Build history of the part. All positions in model axes, mm. Face numbers are marked on the shaded views. A direction names the side the tool comes from. Round coordinates to 2 decimals unless told otherwise and drop trailing zeros. Write each loop counter-clockwise with the first axis right and the second up, starting at its lowest first coordinate (ties: lowest second). Pieces come first, ordered by that corner, then holes. Notation, with made-up numbers: (45, 38) -> (73, 38) arc R21 ccw to (73, 69) -> close; hole circle Ø11 at (-13.5, -8.75). An arc over 180 degrees is marked (long way). Answer in a Markdown table with one row per item.
```python
from build123d import *

# Parameters (mm, degrees)
SKETCH2_W           = 130
SKETCH2_H           = 130
BOSS_EXTRUDE1_DEPTH = 2.5
SKETCH3_W           = 13
SKETCH3_H           = 33
CUT_EXTRUDE1_DEPTH  = 1.2
SKETCH4_W           = 13
SKETCH4_H           = 3
CUT_EXTRUDE2_DEPTH  = 2.3


with BuildPart() as part:
    # Sketch2 → Boss-Extrude1 (new body)
    with BuildSketch(Plane(origin=(0, 0, 0), x_dir=(1, 0, 0), z_dir=(0, 1, 0))):
        Rectangle(SKETCH2_W, SKETCH2_H)
    extrude(amount=BOSS_EXTRUDE1_DEPTH)

    # Sketch3 → Cut-Extrude1 (cut)
    with BuildSketch(Plane(origin=(0, 2.5, 0), x_dir=(1, 0, 0), z_dir=(0, 1, 0))):
        Rectangle(SKETCH3_W, SKETCH3_H)
    extrude(amount=-CUT_EXTRUDE1_DEPTH, mode=Mode.SUBTRACT)

    # Sketch4 → Cut-Extrude2 (cut, through all)
    with BuildSketch(Plane(origin=(0, 1.3, 0), x_dir=(1, 0, 0), z_dir=(0, 1, 0))):
        with Locations((0, 15)):
            Rectangle(SKETCH4_W, SKETCH4_H)
    extrude(amount=-CUT_EXTRUDE2_DEPTH, mode=Mode.SUBTRACT)


solid = part.part
```
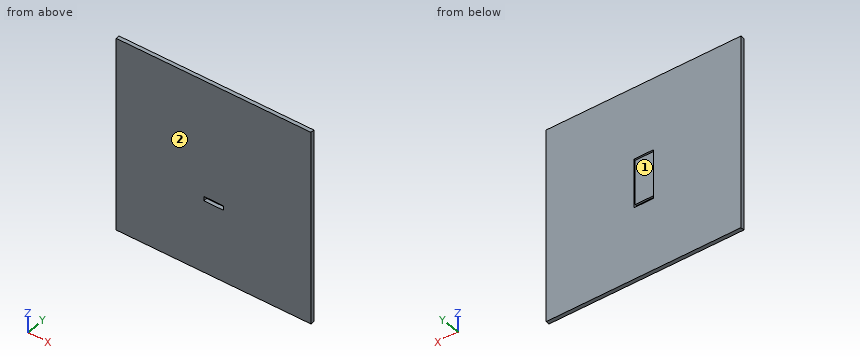
Q1. Which spindle directions (+Z, -Z, +X, -X, +Y, -Y) get a long thin tool onto all of the face, cutting with end or side? Do the marked faces 1 and 2. Say none if no direction does.
A:
| item | result |
|---|---|
| face 1 | +Y |
| face 2 | +Z, -Z, +X, -X, -Y |
Q2. Saw through at A-A on y = 1.85. Write the cut outline in (x, z), plus the area to 3 significant figures.
A:
| item | result |
|---|---|
| outline | (-65, -65) -> (65, -65) -> (65, 65) -> (-65, 65) -> close; hole (-6.5, -16.5) -> (6.5, -16.5) -> (6.5, 16.5) -> (-6.5, 16.5) -> close |
| area | 16,500 mm² |
Q3. Saw through at B-B on z = -12. Write the cut outline in (x, y).
A:
| item | result |
|---|---|
| outline | (-65, 0) -> (65, 0) -> (65, 2.5) -> (6.5, 2.5) -> (6.5, 1.3) -> (-6.5, 1.3) -> (-6.5, 2.5) -> (-65, 2.5) -> close |
Q4. Wall check: line 1 (X direction, y = 2.1, z = 2); line 2 (Y direction, x = -1, z = 14). Give the ranges that are in metal, low to high. Write a range as [from, to].
A:
| item | result |
|---|---|
| line 1 | [-65, -6.5], [6.5, 65] |
| line 2 | [0, 1.3] |
Q5. Drop a flat-ended pin along its axis: P1, Ø4, axis at x = 0.5, z = 8.5, coming from the +Y side. Give the stop position or say it passes through.
A:
| item | result |
|---|---|
| P1 | y = 1.3 |
